Check sheet for the modelled part. Datum: model origin and axes. Units: mm. A direction names the side the tool comes from. Round coordinates to 2 decimals unless told otherwise and drop trailing zeros. Loops run counter-clockwise (first coordinate to the right, second up) from the corner with the lowest first, then second, coordinate; pieces in that order, holes last. Notation, with made-up numbers: M -22.5,87 L 6.5,87 A15 ccw 6.5,110 Z; hole C 64,-25 d1. An arc over 180 degrees is marked long. Write item = value, one per line. Start each with the question number.
(1) Scan lines: L1, parallel to X at y = -0.65, z = 11.5; L2, parallel to X at y = -0.65, z = 8.5; L3, parallel to Z at x = 4, y = -0.8. Record each from-to range of solid material in increasing order. Write a range as from..to.
(2) Cross-section at B-B on z = -13. Record the boundary of the cut face in (x, y).
(3) Set-up check for faces 3 (the face through (3.273, -0.493, 7.97)), 4 (the face through (10, -1, 8)): record each of +Z, -Z, +X, -X, +Y, -Y from which the full face is reachable in a straight line by a thin tool's end or side.
(4) Cross-section at D-D on z = -2. Record the boundary of the cut face in (x, y).
(5) Go/stop test with flat-tipped pins: P1, Ø0.5, axis at x = 22, y = -0.5, coming from the +Z side; P2, Ø0.5, axis at x = 1.5, y = -0.5, coming from the -Z side; P3, Ø0.5, axis at y = -0.5, z = -4, coming from the -X side. Record where each tip stops, or that it passes through.
(6) Cross-section at A-A on x = 21.5. Record the boundary of the cut face in (y, z).
(7) Mould release check, pull along X, two halves, no side actions. Record for faces 1 (the face through (10, 0, 8)), 2 (the face through (23.273, -0.493, 7.97)): pulls with the +X half, pulls with the -X half, needs draft (parallel to the pull), parting line crosses it, or undercut.
(8) Cross-section at C-C on y = -0.4. State how many separate pieces and enclosed holes the cut face has, plus the area to 3 significant figures.
from build123d import *
from build123d.topology import SkipClean

# Parameters (mm, degrees)
L_U_BR_IST_W               = 55
L_U_BR_IST_H               = 55
AUFSATZ_LIN_GK_DEPTH       = 1
SCHNITT_LIN_S1_DEPTH       = 2
SCHNITT_LIN_S2_DEPTH       = 2
SCHNITT_LIN_S3_DEPTH       = 2
SCHNITT_LIN_S4_DEPTH       = 2
LIN_MUSTER_S1_COUNT        = 2
LIN_MUSTER_S1_PITCH        = 20
LIN_MUSTER_S1_COUNT_DIR2   = 3
LIN_MUSTER_S1_PITCH_DIR2   = 20
LIN_MUSTER_S2_COUNT        = 2
LIN_MUSTER_S2_PITCH        = 20
LIN_MUSTER_S3_COUNT        = 2
LIN_MUSTER_S3_PITCH        = 20
SPIEGELN_S4_Z_COPY_1_DEPTH = 2
SPIEGELN_S2_COPY_1_DEPTH   = 2
SPIEGELN_S3_COPY_1_DEPTH   = 2
SPIEGELN_S3_COPY_2_DEPTH   = 2


with BuildPart() as part:
    # L_ u Br Ist → Aufsatz-Lin_GK (new body)
    with BuildSketch(Plane(origin=(0, 0, 0), x_dir=(1, 0, 0), z_dir=(0, 1, 0))):
        with Locations((10.772595927, -7.907273432)):
            Rectangle(L_U_BR_IST_W, L_U_BR_IST_H)
    extrude(amount=-AUFSATZ_LIN_GK_DEPTH)

    # Sketch S1 → Schnitt-Lin_S1 (cut, through all)
    with BuildSketch(Plane(origin=(0, 0, 0), x_dir=(1, 0, 0), z_dir=(0, 1, 0))):
        with BuildLine():
            Line((-2.613025796, 7.092726568), (4.158217649, 7.092726568))
            ThreePointArc((4.158217649, 7.092726568), (4.600159387, 7.358872981), (4.571616291, 7.873976568))
            ThreePointArc((4.571616291, 7.873976568), (3.272595927, 12.092726568), (4.571616291, 16.311476568))
            ThreePointArc((4.571616291, 16.311476568), (4.600159387, 16.826580155), (4.158217649, 17.092726568))
            Line((4.158217649, 17.092726568), (-2.613025796, 17.092726568))
            ThreePointArc((-2.613025796, 17.092726568), (-3.054967534, 16.826580155), (-3.026424438, 16.311476568))
            ThreePointArc((-3.026424438, 16.311476568), (-1.727404073, 12.092726568), (-3.026424438, 7.873976568))
            ThreePointArc((-3.026424438, 7.873976568), (-3.054967534, 7.358872981), (-2.613025796, 7.092726568))
        make_face()
    schnitt_lin_s1 = extrude(amount=-SCHNITT_LIN_S1_DEPTH, mode=Mode.SUBTRACT)

    # Sketch S2 → Schnitt-Lin_S2 (cut, through all)
    with BuildSketch(Plane(origin=(0, 0, 0), x_dir=(1, 0, 0), z_dir=(0, 1, 0))):
        with BuildLine():
            Line((-14.817574017, -2.719804872), (-14.817574017, 6.905258008))
            ThreePointArc((-14.817574017, 6.905258008), (-14.848363078, 7.07800376), (-14.936938396, 7.229474793))
            ThreePointArc((-14.936938396, 7.229474793), (-16.26556816, 9.501540297), (-16.727404073, 12.092726568))
            Line((-16.727404073, 12.092726568), (-16.727404073, -7.907273432))
            ThreePointArc((-16.727404073, -7.907273432), (-16.26556816, -5.316087161), (-14.936938396, -3.044021657))
            ThreePointArc((-14.936938396, -3.044021657), (-14.848363078, -2.892550624), (-14.817574017, -2.719804872))
        make_face()
    schnitt_lin_s2 = extrude(amount=-SCHNITT_LIN_S2_DEPTH, mode=Mode.SUBTRACT)

    # Sketch S3 → Schnitt-Lin_S3 (cut, through all)
    with BuildSketch(Plane(origin=(0, 0, 0), x_dir=(1, 0, 0), z_dir=(0, 1, 0))):
        with BuildLine():
            Line((-3.026424438, 16.311476568), (4.571616291, 16.311476568))
            ThreePointArc((4.571616291, 16.311476568), (7.264792127, 18.721852642), (10.772595927, 19.592726568))
            Line((10.772595927, 19.592726568), (-9.227404073, 19.592726568))
            ThreePointArc((-9.227404073, 19.592726568), (-5.719600273, 18.721852642), (-3.026424438, 16.311476568))
        make_face()
    schnitt_lin_s3 = extrude(amount=-SCHNITT_LIN_S3_DEPTH, mode=Mode.SUBTRACT)

    # Sketch S4 → Schnitt-Lin_S4 (cut, through all)
    with SkipClean():  # keep this step's faces unmerged: merging them makes the solid invalid here
        with BuildSketch(Plane(origin=(0, 0, 0), x_dir=(1, 0, 0), z_dir=(0, 1, 0))):
            with BuildLine():
                Line((-16.727404073, 12.092726568), (-16.727404073, 19.592726568))
                Line((-16.727404073, 19.592726568), (-9.227404073, 19.592726568))
                ThreePointArc((-9.227404073, 19.592726568), (-14.530704932, 17.396027427), (-16.727404073, 12.092726568))
            make_face()
        schnitt_lin_s4 = extrude(amount=-SCHNITT_LIN_S4_DEPTH, mode=Mode.SUBTRACT)

    # Lin Muster_S1: Schnitt-Lin_S1 2 × 3
    with SkipClean():  # keep this step's faces unmerged: merging them makes the solid invalid here
        with Locations(*[(i * LIN_MUSTER_S1_PITCH, 0, j * LIN_MUSTER_S1_PITCH_DIR2) for i in range(LIN_MUSTER_S1_COUNT) for j in range(LIN_MUSTER_S1_COUNT_DIR2) if (i, j) != (0, 0)]):
            add(schnitt_lin_s1, mode=Mode.SUBTRACT)

    # Lin Muster_S2: Schnitt-Lin_S2 ×2
    with SkipClean():  # keep this step's faces unmerged: merging them makes the solid invalid here
        with Locations(*[(0, 0, i * LIN_MUSTER_S2_PITCH) for i in range(1, LIN_MUSTER_S2_COUNT)]):
            add(schnitt_lin_s2, mode=Mode.SUBTRACT)

    # Lin Muster_S3: Schnitt-Lin_S3 ×2
    with SkipClean():  # keep this step's faces unmerged: merging them makes the solid invalid here
        with Locations(*[(i * LIN_MUSTER_S3_PITCH, 0, 0) for i in range(1, LIN_MUSTER_S3_COUNT)]):
            add(schnitt_lin_s3, mode=Mode.SUBTRACT)

    # Spiegeln_S4 X: Schnitt-Lin_S4 across plane
    with SkipClean():  # keep this step's faces unmerged: merging them makes the solid invalid here
        add(schnitt_lin_s4.mirror(Plane.ZY.offset(-10.772595927)), mode=Mode.SUBTRACT)

    # Spiegeln_S4 Z: Schnitt-Lin_S4 across plane
    with SkipClean():  # keep this step's faces unmerged: merging them makes the solid invalid here
        add(schnitt_lin_s4.mirror(Plane.XY.offset(7.907273432)), mode=Mode.SUBTRACT)

    # Spiegeln_S4 Z copy 1 sketch → Spiegeln_S4 Z copy 1 (cut, through all)
    with SkipClean():  # keep this step's faces unmerged: merging them makes the solid invalid here
        with BuildSketch(Plane(origin=(21.545191853, 0, 15.814546864), x_dir=(-1, 0, 0), z_dir=(0, 1, 0))):
            with BuildLine():
                Line((-16.727404073, 12.092726568), (-16.727404073, 19.592726568))
                Line((-16.727404073, 19.592726568), (-9.227404073, 19.592726568))
                ThreePointArc((-9.227404073, 19.592726568), (-14.530704932, 17.396027427), (-16.727404073, 12.092726568))
            make_face()
        extrude(amount=-SPIEGELN_S4_Z_COPY_1_DEPTH, mode=Mode.SUBTRACT)

    # Spiegeln_S2: Schnitt-Lin_S2 across plane
    with SkipClean():  # keep this step's faces unmerged: merging them makes the solid invalid here
        add(schnitt_lin_s2.mirror(Plane.ZY.offset(-10.772595927)), mode=Mode.SUBTRACT)

    # Spiegeln_S2 copy 1 sketch → Spiegeln_S2 copy 1 (cut, through all)
    with SkipClean():  # keep this step's faces unmerged: merging them makes the solid invalid here
        with BuildSketch(Plane(origin=(21.545191853, 0, 20), x_dir=(-1, 0, 0), z_dir=(0, 1, 0))):
            with BuildLine():
                Line((-14.817574017, 2.719804872), (-14.817574017, -6.905258008))
                ThreePointArc((-14.817574017, -6.905258008), (-14.848363078, -7.07800376), (-14.936938396, -7.229474793))
                ThreePointArc((-14.936938396, -7.229474793), (-16.26556816, -9.501540297), (-16.727404073, -12.092726568))
                Line((-16.727404073, -12.092726568), (-16.727404073, 7.907273432))
                ThreePointArc((-16.727404073, 7.907273432), (-16.26556816, 5.316087161), (-14.936938396, 3.044021657))
                ThreePointArc((-14.936938396, 3.044021657), (-14.848363078, 2.892550624), (-14.817574017, 2.719804872))
            make_face()
        extrude(amount=-SPIEGELN_S2_COPY_1_DEPTH, mode=Mode.SUBTRACT)

    # Spiegeln_S3 copy 1 sketch → Spiegeln_S3 copy 1 (cut, through all)
    with SkipClean():  # keep this step's faces unmerged: merging them makes the solid invalid here
        with BuildSketch(Plane(origin=(20, 0, 15.814546864), x_dir=(1, 0, 0), z_dir=(0, 1, 0))):
            with BuildLine():
                Line((-3.026424438, -16.311476568), (4.571616291, -16.311476568))
                ThreePointArc((4.571616291, -16.311476568), (7.264792127, -18.721852642), (10.772595927, -19.592726568))
                Line((10.772595927, -19.592726568), (-9.227404073, -19.592726568))
                ThreePointArc((-9.227404073, -19.592726568), (-5.719600273, -18.721852642), (-3.026424438, -16.311476568))
            make_face()
        extrude(amount=-SPIEGELN_S3_COPY_1_DEPTH, mode=Mode.SUBTRACT)

    # Spiegeln_S3 copy 2 sketch → Spiegeln_S3 copy 2 (cut, through all)
    with SkipClean():  # keep this step's faces unmerged: merging them makes the solid invalid here
        with BuildSketch(Plane(origin=(0, 0, 15.814546864), x_dir=(1, 0, 0), z_dir=(0, 1, 0))):
            with BuildLine():
                Line((-3.026424438, -16.311476568), (4.571616291, -16.311476568))
                ThreePointArc((4.571616291, -16.311476568), (7.264792127, -18.721852642), (10.772595927, -19.592726568))
                Line((10.772595927, -19.592726568), (-9.227404073, -19.592726568))
                ThreePointArc((-9.227404073, -19.592726568), (-5.719600273, -18.721852642), (-3.026424438, -16.311476568))
            make_face()
        extrude(amount=-SPIEGELN_S3_COPY_2_DEPTH, mode=Mode.SUBTRACT)


solid = part.part
Result:
q1.L1 = -15.81..-2.64, 4.19..17.36, 24.19..37.36
q1.L2 = -16.7..-1.75, 3.3..18.25, 23.3..38.25
q1.L3 = -15.31..-8.87, -7.09..2.91, 4.69..11.13, 12.91..22.91, 24.69..31.13
q2.outline = M -16.67,-1 L -1.78,-1 L -1.78,0 L -16.67,0 Z; M 3.33,-1 L 18.22,-1 L 18.22,0 L 3.33,0 Z; M 23.33,-1 L 38.22,-1 L 38.22,0 L 23.33,0 Z
q3.face_3 = +Y, -Y
q3.face_4 = +Z, -Z, +X, -X, -Y
q4.outline = M -14.82,-1 L 36.36,-1 L 36.36,0 L -14.82,0 Z
q5.P1 = 22.91
q5.P2 = -7.09
q5.P3 = -14.82
q6.outline = M -1,-7.09 L 0,-7.09 L 0,2.91 L -1,2.91 Z; M -1,12.91 L 0,12.91 L 0,22.91 L -1,22.91 Z
q7.face_1 = needs draft
q7.face_2 = undercut
q8.separate_pieces = 1
q8.enclosed_holes = 2
q8.area = 2,390 mm^2
